Autodesk Inventor part; units mm, degrees
ref_plane "YZ Plane" through (0, 0, 0) normal (1, 0, 0) x (0, 1, 0)
ref_plane "XZ Plane" through (0, 0, 0) normal (0, 1, 0) x (-1, 0, 0)
ref_plane "XY Plane" through (0, 0, 0) normal (0, 0, 1) x (1, 0, 0)
sketch "Esboço1" plane through (0, 0, 0) normal (0, 0, 1) x (1, 0, 0)
  line L0 (-13, 11.5) -> (13, 11.5)
  line L1 (13, 11.5) -> (13, -11.5)
  line L2 (13, -11.5) -> (-13, -11.5)
  line L3 (-13, -11.5) -> (-13, 11.5)
  line L4 (-13, 11.5) -> (13, -11.5) construction
  line L5 (13, 11.5) -> (-13, -11.5) construction
  point P0 (0, 0)
  dimension "d0" = 26
  dimension "d1" = 23
extrude "Extrusão1" add sketch "Esboço1" along normal blind 2
chamfer "Chanfro1" distance 2 angle 45 4 edges at (-13, 11.5, 1) (-13, -11.5, 1) (13, 11.5, 1) (13, -11.5, 1)
sketch "Esboço2" plane through (0, 0, 2) normal (0, 0, 1) x (1, 0, 0)
  line L0 (-10.75, 6.8) -> (10.75, 6.8)
  line L1 (10.75, 6.8) -> (10.75, 9.3)
  line L2 (10.75, 9.3) -> (-10.75, 9.3)
  line L3 (-10.75, 9.3) -> (-10.75, 6.8)
  line L4 (-10.75, 6.8) -> (10.75, 9.3) construction
  line L5 (10.75, 6.8) -> (-10.75, 9.3) construction
  line L6 (11, 11.5) -> (-11, 11.5)
  line L7 (-13, 9.5) -> (-13, -9.5)
  line L8 (0, 0) -> (3.5372, 0) construction
  line L9 (-10.75, -6.8) -> (10.75, -6.8)
  line L10 (10.75, -6.8) -> (10.75, -9.3)
  line L11 (10.75, -9.3) -> (-10.75, -9.3)
  line L12 (-10.75, -9.3) -> (-10.75, -6.8)
  line L13 (-10.75, -6.8) -> (10.75, -9.3) construction
  line L14 (10.75, -6.8) -> (-10.75, -9.3) construction
  point P0 (0, 8.05)
  point P1 (0, -8.05)
  dimension "d7" = 21.5
  dimension "d8" = 2.5
  dimension "d9" = 2.2
  dimension "d10" = 2.25
extrude "Extrusão2" add sketch "Esboço2" along normal blind 2
chamfer "Chanfro2" distance 2 angle 45 4 edges at (-10.75, 9.3, 3) (10.75, 9.3, 3) (10.75, -9.3, 3) (-10.75, -9.3, 3)
sketch "Esboço3" plane through (0, 0, 2) normal (0, 0, 1) x (1, 0, 0)
  line L0 (-1, -2.8) -> (1, -2.8)
  line L1 (1, -2.8) -> (1, -4.8)
  line L2 (1, -4.8) -> (-1, -4.8)
  line L3 (-1, -4.8) -> (-1, -2.8)
  line L4 (-1, -2.8) -> (1, -4.8) construction
  line L5 (1, -2.8) -> (-1, -4.8) construction
  line L6 (-10.75, -6.8) -> (10.75, -6.8)
  line L7 (13, -9.5) -> (13, 9.5)
  point P0 (0, 0)
  point P1 (0, -3.8)
  dimension "d16" = 2
  dimension "d17" = 2
  dimension "d18" = 2
  dimension "d19" = 12
extrude "Extrusão3" cut sketch "Esboço3" against normal blind 10
properties part number "TampaEletronica"
Geometry: final body of the model. Coordinates: model frame, mm. A direction names the side the tool comes from. Give positions to 0.01 mm unless a question says otherwise; leave off trailing zeros. Loops run counter-clockwise (first coordinate to the right, second up) from the corner with the lowest first, then second, coordinate; pieces in that order, holes last. Notation, with made-up numbers: M 20.25,15.25 L 37.25,15.25 A28 ccw 37.25,45.25 Z; hole C 46.5,24.25 d4. An arc over 180 degrees is marked long. Put each result on its own line as item: value. Start each with the question number.
1) Pull-direction query (X, two-part tool) for faces 1 (the flat face through (0, -6.8, 3)), 2 (the flat face through (1, -4, 1)), 3 (the flat face through (13, 0, 1)); classes: pulls with the +X half, pulls with the -X half, needs draft (parallel to the pull), parting line crosses it, or undercut.
2) Cut plane C-C (z = 1.55). Output: boundary loops of the cut face in (x, y).
3) Cut plane B-B (y = -3.5). Output: boundary loops of the cut face in (x, z).
4) Cut plane D-D (x = 0.5). Output: boundary loops of the cut face in (y, z).
5) Cut plane A-A (z = 3.3). Output: boundary loops of the cut face in (x, y).
6) Ray query, line 1 along Y through (x, z) = (6.25, 3.1); line 2 along Y through (x, z) = (0.25, 0.6); line 3 along Z through (x, y) = (-4.5, 4.5). Return the intervals inside material, ascending.
7) Contact query for flat-ended pins moving along their axis: pin 1 (1 mm diameter, centred on x = 0.5, z = 3, fed in from +Y); pin 2 (0.6 mm diameter, centred on x = -0.5, z = 3, fed in from -Y); pin 3 (8 mm diameter, centred on x = -9, y = 0.5, fed in from +Z). Output: stop coordinate, or through.
8) Access query for faces 4 (the flat face through (9.74, 8.31, 3.01)), 5 (the flat face through (0, 9.3, 3)), 6 (the flat face through (9.76, -8.29, 3.01)). Directions: +Z, -Z, +X, -X, +Y, -Y. A direction counts if a zero-diameter tool reaches every point of the face in a straight line with its end or side. Return the directions, or none.
Verdict:
1. face 1: needs draft
1. face 2: undercut
1. face 3: pulls with the +X half
2. outline: M -13,-9.5 L -11,-11.5 L 11,-11.5 L 13,-9.5 L 13,9.5 L 11,11.5 L -11,11.5 L -13,9.5 Z; hole M -1,-4.8 L 1,-4.8 L 1,-2.8 L -1,-2.8 Z
3. outline: M -13,0 L -1,0 L -1,2 L -13,2 Z; M 1,0 L 13,0 L 13,2 L 1,2 Z
4. outline: M -11.5,0 L -4.8,0 L -4.8,2 L -6.8,2 L -6.8,4 L -9.3,4 L -9.3,2 L -11.5,2 Z; M -2.8,0 L 11.5,0 L 11.5,2 L 9.3,2 L 9.3,4 L 6.8,4 L 6.8,2 L -2.8,2 Z
5. outline: M -10.75,-7.3 L -8.75,-9.3 L 8.75,-9.3 L 10.75,-7.3 L 10.75,-6.8 L -10.75,-6.8 Z; M -10.75,6.8 L 10.75,6.8 L 10.75,7.3 L 8.75,9.3 L -8.75,9.3 L -10.75,7.3 Z
6. line 1: -9.3 to -6.8, 6.8 to 9.3
6. line 2: -11.5 to -4.8, -2.8 to 11.5
6. line 3: 0 to 2
7. pin 1: y = 9.3
7. pin 2: y = -9.3
7. pin 3: z = 2
8. face 4: +Z, +X, +Y
8. face 5: +Z, +X, -X, +Y
8. face 6: +Z, +X, -Y
